```python
from build123d import *

# Parameters (mm, degrees)
SKETCH1_W               = 19.5
SKETCH1_H               = 10
BOSS_EXTRUDE1_DEPTH     = 4
SKETCH2_W               = 9
SKETCH2_H               = 5.5
CUT_EXTRUDE1_DEPTH      = 2.7
SKETCH3_W               = 3.2
SKETCH3_H               = 3.9
CUT_EXTRUDE2_DEPTH      = 12.664583147
SKETCH4_W               = 1.747901038
SKETCH4_H               = 5.5
CUT_EXTRUDE3_DEPTH      = 12.285056491
CHAMFER2_SIZE           = 1
SKETCH5_W               = 10
SKETCH5_H               = 4
BOSS_EXTRUDE2_DEPTH     = 2
SKETCH6_W               = 1.747077863
SKETCH6_H               = 5.5
BOSS_EXTRUDE3_DEPTH     = 1.5
BOSS_EXTRUDE4_DEPTH     = 2
BOSS_EXTRUDE5_REACH     = 16.109
SKETCH9_W               = 3.657403566
SKETCH9_H               = 0.3
SKETCH10_W              = 5.81497097
SKETCH10_H              = 2.25
SKETCH10_W_2            = 5.452409629
BOSS_EXTRUDE6_DEPTH     = 2
CUT_EXTRUDE4_DEPTH      = 3.8
CUT_EXTRUDE4_DEPTH_BACK = 1
SKETCH12_W              = 1.656525066
SKETCH12_H              = 10


with BuildPart() as part:
    # Sketch1 → Boss-Extrude1 (new body)
    with BuildSketch(Plane(origin=(0, 0, 0), x_dir=(1, 0, 0), z_dir=(0, 1, 0))):
        Rectangle(SKETCH1_W, SKETCH1_H)
    extrude(amount=BOSS_EXTRUDE1_DEPTH)

    # Sketch2 → Cut-Extrude1 (cut)
    with BuildSketch(Plane(origin=(0, 4, 0), x_dir=(1, 0, 0), z_dir=(0, 1, 0))):
        with Locations((5.25, 0)):
            Rectangle(SKETCH2_W, SKETCH2_H)
    extrude(amount=-CUT_EXTRUDE1_DEPTH, mode=Mode.SUBTRACT)

    # Sketch3 → Cut-Extrude2 (cut, through all)
    with BuildSketch(Plane(origin=(0, 4, 0), x_dir=(1, 0, 0), z_dir=(0, 1, 0))):
        with Locations((-8.15, 3.05)):
            Rectangle(SKETCH3_W, SKETCH3_H)
        with Locations((-8.15, -3.05)):
            Rectangle(SKETCH3_W, SKETCH3_H)
    extrude(amount=-CUT_EXTRUDE2_DEPTH, mode=Mode.SUBTRACT)

    # Sketch4 → Cut-Extrude3 (cut, through all)
    with BuildSketch(Plane(origin=(0, 1.3, 0), x_dir=(1, 0, 0), z_dir=(0, 1, 0))):
        with Locations((1.623950519, 0)):
            Rectangle(SKETCH4_W, SKETCH4_H)
    extrude(amount=-CUT_EXTRUDE3_DEPTH, mode=Mode.SUBTRACT)

    # Chamfer2
    chamfer2_edges = [part.edges().sort_by_distance(p)[0] for p in [
        (2.497901038, 1.3, 0),
    ]]
    chamfer(chamfer2_edges, length=CHAMFER2_SIZE)

    # Sketch5 → Boss-Extrude2 (add)
    with BuildSketch(Plane(origin=(9.75, 0, 0), x_dir=(0, 0, -1), z_dir=(1, 0, 0))):
        with Locations((0, 2)):
            Rectangle(SKETCH5_W, SKETCH5_H)
    extrude(amount=BOSS_EXTRUDE2_DEPTH)

    # Sketch6 → Boss-Extrude3 (add)
    with BuildSketch(Plane(origin=(0, 1.3, 0), x_dir=(1, 0, 0), z_dir=(0, 1, 0))):
        with Locations((8.876461068, 0)):
            Rectangle(SKETCH6_W, SKETCH6_H)
    extrude(amount=BOSS_EXTRUDE3_DEPTH)

    # Sketch7 → Boss-Extrude4 (add)
    with BuildSketch(Plane(origin=(0, 4, 0), x_dir=(1, 0, 0), z_dir=(0, 1, 0))):
        Polygon((2.760699465, 2.75), (2.760699465, 5), (11.75, 5), (11.75, -5), (2.760699465, -5), (2.760699465, -2.75), (9.75, -2.75), (9.75, 2.75), align=None)
    extrude(amount=BOSS_EXTRUDE4_DEPTH)

    # Sketch9 → Boss-Extrude5 (add, up to next)
    with BuildSketch(Plane(origin=(0, 6, 0), x_dir=(1, 0, 0), z_dir=(0, 1, 0)), mode=Mode.PRIVATE) as boss_extrude5_sk1:
        with Locations((7.921298217, 2.6)):
            Rectangle(SKETCH9_W, SKETCH9_H)
    boss_extrude5_tool1 = extrude(boss_extrude5_sk1.sketch, amount=-BOSS_EXTRUDE5_REACH, mode=Mode.PRIVATE) - part.part
    # Sketch9 → Boss-Extrude5 (add, up to next)
    with BuildSketch(Plane(origin=(0, 6, 0), x_dir=(1, 0, 0), z_dir=(0, 1, 0)), mode=Mode.PRIVATE) as boss_extrude5_sk2:
        with Locations((7.921298217, -2.6)):
            Rectangle(SKETCH9_W, SKETCH9_H)
    boss_extrude5_tool2 = extrude(boss_extrude5_sk2.sketch, amount=-BOSS_EXTRUDE5_REACH, mode=Mode.PRIVATE) - part.part
    add(boss_extrude5_tool1.solids().sort_by_distance((7.921298, 6, -2.6))[0])
    add(boss_extrude5_tool2.solids().sort_by_distance((7.921298, 6, 2.6))[0])

    # Sketch10 → Boss-Extrude6 (add)
    with BuildSketch(Plane(origin=(0, 4, 0), x_dir=(1, 0, 0), z_dir=(0, 1, 0))):
        with Locations((-3.642514515, 3.875)):
            Rectangle(SKETCH10_W, SKETCH10_H)
        with Locations((-3.823795186, -3.875)):
            Rectangle(SKETCH10_W_2, SKETCH10_H)
    extrude(amount=BOSS_EXTRUDE6_DEPTH)

    # Sketch12 → Cut-Extrude4 (cut, two sides: drawn at the far end of the back side and taken through both)
    with BuildSketch(Plane(origin=(0, 4, 0), x_dir=(1, 0, 0), z_dir=(0, 1, 0)).offset(-CUT_EXTRUDE4_DEPTH_BACK)):
        with Locations((-0.269327838, 0)):
            Rectangle(SKETCH12_W, SKETCH12_H)
    extrude(amount=CUT_EXTRUDE4_DEPTH + CUT_EXTRUDE4_DEPTH_BACK, mode=Mode.SUBTRACT)


solid = part.part
```
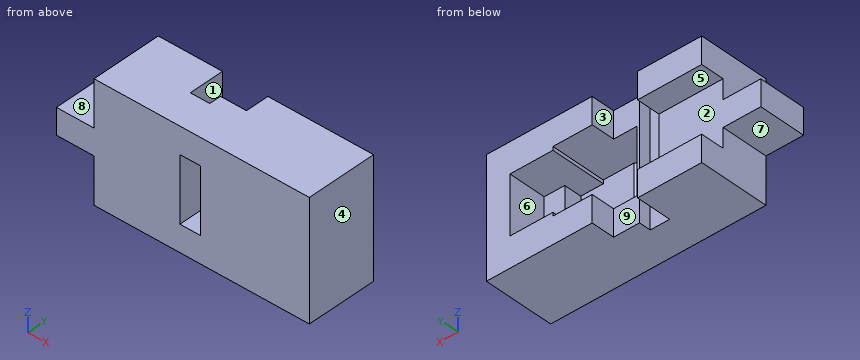
Part model, mm, in its own coordinate system. Face numbers are marked on the shaded views. A direction names the side the tool comes from. Give positions to 0.01 mm unless a question says otherwise; leave off trailing zeros. Loops run counter-clockwise (first coordinate to the right, second up) from the corner with the lowest first, then second, coordinate; pieces in that order, holes last. Notation, with made-up numbers: M -34.5,-33 L 24.5,-33 A18 cw 24.5,-20 Z; hole C -25.75,13.5 d3. An arc over 180 degrees is marked long. Return JSON: item names as keys, results as strings.
1) 3-axis set-ups, long thin cutter, end or side, ignore diameter. For the marked faces 5, 6, 7, 8 and 9: which of +Z, -Z, +X, -X, +Y, -Y reach the whole face in a straight line?
Calculated:
{"face 5": "-X, +Y", "face 6": "+Y", "face 7": "-Z, -X, +Y, -Y", "face 8": "+Z, -X, +Y, -Y", "face 9": "+Z, -Z, +Y"}
2) Drill centre lines: line 1 (X direction, y = 3.45, z = -2.25); line 2 (Z direction, x = 3.5, y = 3.7); line 3 (Z direction, x = 7.25, y = 2.75). Where is each one in solid material? Low to high.
Calculated:
{"line 1": "x = -6.55 to -1.1, 0.56 to 0.75, 9.75 to 11.75", "line 2": "z = -5 to -2.75, 2.75 to 5", "line 3": "z = -5 to -2.45, 2.45 to 5"}
3) Saw through at C-C, the plane x = 8.5. List the corners of the cut face in (y, z), then the cut area to 3 significant figures.
Calculated:
{"outline": "M 0,-5 L 6,-5 L 6,-2.45 L 2.8,-2.45 L 2.8,2.45 L 6,2.45 L 6,5 L 0,5 Z", "area": "44.3 mm2"}
4) Saw through at B-B, the plane y = 4.75. List the corners of the cut face in (x, z).
Calculated:
{"outline": "M -6.55,-5 L -1.1,-5 L -1.1,-2.75 L -6.55,-2.75 Z; M -6.55,2.75 L -1.1,2.75 L -1.1,5 L -6.55,5 Z; M 2.76,-5 L 11.75,-5 L 11.75,5 L 2.76,5 L 2.76,2.75 L 6.09,2.75 L 6.09,2.45 L 9.75,2.45 L 9.75,-2.45 L 6.09,-2.45 L 6.09,-2.75 L 2.76,-2.75 Z"}
5) Saw through at A-A, the plane z = -2. List the corners of the cut face in (x, y).
Calculated:
{"outline": "M -6.55,0 L 0.75,0 L 0.75,4 L 0.56,4 L 0.56,3 L -1.1,3 L -1.1,4 L -6.55,4 Z; M 2.5,0 L 11.75,0 L 11.75,6 L 9.75,6 L 9.75,2.8 L 8,2.8 L 8,1.3 L 3.5,1.3 L 2.5,0.3 Z"}
6) Saw through at D-D, the plane z = 3.25. List the corners of the cut face in (x, y), then the cut area to 3 significant figures.
Calculated:
{"outline": "M -6.55,0 L 11.75,0 L 11.75,6 L 2.76,6 L 2.76,4 L 0.56,4 L 0.56,3 L -1.1,3 L -1.1,6 L -6.55,6 Z", "area": "100 mm2"}
7) Pull direction X, two halves, no side cores. Call the marked faces 1, 2, 3 and 4: released by +X, released by -X, zero draft, split by the parting line, or undercut.
Calculated:
{"face 1": "undercut", "face 2": "zero draft", "face 3": "undercut", "face 4": "released by +X"}
8) Flat gauge pins, fed straight in: pin 1 Ø1.8 at (x, z) = (1.5, 1.5) entering from +Y; pin 2 Ø1 at (y, z) = (5, 4) entering from -X; pin 3 Ø1 at (x, y) = (-8, 1) entering from -Z. Where does each tip first touch, or does it go through?
Calculated:
{"pin 1": "stops at y = 4", "pin 2": "stops at x = -6.55", "pin 3": "stops at z = -1.1"}
